Geometry check sheet. Reference: the model listing, model coordinates, mm. A direction names the side the tool comes from. Coordinates: 2 decimals unless noted, no trailing zeros. Write each loop counter-clockwise with the first axis right and the second up, starting at its lowest first coordinate (ties: lowest second). Pieces come first, ordered by that corner, then holes. Notation, with made-up numbers: (26.5, 34.25) -> (30.5, 34.25) arc R10 cw to (30.5, 39.25) -> close; hole circle Ø11 at (60.5, -10). An arc over 180 degrees is marked (long way). Answer in a Markdown table with one row per item. Add a question column.
1. Cross-section at D-D on z = -115. Record the cut outline in (x, y), and give its area (3 significant figures).
2. Mould release check, pull along X, two halves, no side actions. Record for faces 6 (the cylindrical face through (17.27, 0.2, -10.09)), 7 (the flat face through (50.411, 0.197, 33.724)), 8 (the flat face through (-54.411, 0.197, 26.796)): pulls with the +X half, pulls with the -X half, needs draft (parallel to the pull), parting line crosses it, or undercut.
3. Set-up check for faces 1 (the cylindrical face through (-0.49, 0.2, -129.99)), 2 (the flat face through (-51.06, 0.2, 34.1)), 3 (the cylindrical face through (-6.355, 0.203, -23.574)), 4 (the cylindrical face through (-23.762, 0.203, 6.527)), 5 (the cylindrical face through (5.805, 0.203, -96.985)): record each of +Z, -Z, +X, -X, +Y, -Y from which the full face is reachable in a straight line by a thin tool's end or side.
4. Cross-section at C-C on x = 0. Record the cut outline in (y, z), and give its area (3 significant figures).
5. Cross-section at A-A on z = 52.5. Record the cut outline in (x, y).
6. Scan lines: L1, parallel to X at y = 0.05, z = -88; L2, parallel to X at y = 0.15, z = 47; L3, parallel to X at y = 0.1, z = 48.5. Record each from-to range of solid material in increasing order. Write a range as from..to.
7. Cross-section at B-B on y = 0.3. Record the cut outline in (x, z), and give its area (3 significant figures).
Autodesk Fusion 360 part; units mm, degrees
sketch "Sketch1" plane through (0, 0, 0) normal (0, 1, 0) x (1, 0, 0)
  line L0 (0, 130) -> (-112.5833, -65) construction
  line L1 (-112.5833, -65) -> (112.5833, -65) construction
  line L2 (112.5833, -65) -> (0, 130) construction
  line L3 (0, 0) -> (0, 130) construction
  line L4 (0, 0) -> (-112.5833, -65) construction
  line L5 (0, 0) -> (112.5833, -65) construction
  circle A0 centre (0, 115) radius 15
  circle A1 centre (-99.5929, -57.5) radius 15
  circle A2 centre (99.5929, -57.5) radius 15
  circle A3 centre (0, 0) radius 20
  line L6 (-4, 19.5959) -> (4, 19.5959) construction
  line L7 (4, 19.5959) -> (4, 100.5432)
  line L8 (4, 100.5432) -> (-4, 100.5432) construction
  line L9 (-4, 100.5432) -> (-4, 19.5959)
  line L10 (-85.0729, -53.7357) -> (-14.9706, -13.2621)
  line L11 (-18.9706, -6.3339) -> (-89.0729, -46.8075)
  line L12 (89.0729, -46.8075) -> (18.9706, -6.3339)
  line L13 (14.9706, -13.2621) -> (85.0729, -53.7357)
  point P0 (0, 100.5432)
  point P1 (0, 19.5959)
  dimension "d1" = 130
  dimension "d2" = 30
  dimension "d4" = 360
  dimension "d5" = 40
  dimension "d6" = 8
  dimension "d8" = 360
extrude "Extrude1" add sketch "Sketch1" along normal blind 0.4
fillet "Fillet1" radius 24 12 edges at (-4, 0.2, -100.5432) (4, 0.2, -100.5432) (-4, 0.2, -19.5959) (4, 0.2, -19.5959) (-18.9706, 0.2, 6.3339) (-14.9706, 0.2, 13.2621) (14.9706, 0.2, 13.2621) (18.9706, 0.2, 6.3339) (85.0729, 0.2, 53.7357) (89.0729, 0.2, 46.8075) (-89.0729, 0.2, 46.8075) (-85.0729, 0.2, 53.7357)
Results found:
| question | item | result |
|---|---|---|
| 1 | outline | (-15, 0) -> (15, 0) -> (15, 0.4) -> (-15, 0.4) -> close |
| 1 | area | 12.0 mm^2 |
| 2 | face 6 | pulls with the +X half |
| 2 | face 7 | undercut |
| 2 | face 8 | pulls with the -X half |
| 3 | face 1 | +Y, -Y |
| 3 | face 2 | +Z, +Y, -Y |
| 3 | face 3 | -X, +Y, -Y |
| 3 | face 4 | -Z, -X, +Y, -Y |
| 3 | face 5 | +X, +Y, -Y |
| 4 | outline | (0, -130) -> (0.4, -130) -> (0.4, 20) -> (0, 20) -> close |
| 4 | area | 60.0 mm^2 |
| 5 | outline | (-113.74, 0) -> (-80.26, 0) -> (-80.26, 0.4) -> (-113.74, 0.4) -> close; (80.26, 0) -> (113.74, 0) -> (113.74, 0.4) -> (80.26, 0.4) -> close |
| 6 | L1 | x = -4..4 |
| 6 | L2 | x = -110.31..-73.41, 73.41..110.31 |
| 6 | L3 | x = -111.59..-75.83, 75.83..111.59 |
| 7 | outline | (-95.93, 42.95) arc R24 cw to (-78.08, 40.46) -> (-31.39, 13.51) arc R24 cw to (-19.72, -3.31) arc R20 ccw to (-12.73, -15.43) arc R24 cw to (-4, -33.94) -> (-4, -87.85) arc R24 cw to (-10.77, -104.56) arc R15 ccw (long way) to (10.77, -104.56) arc R24 cw to (4, -87.85) -> (4, -33.94) arc R24 cw to (12.73, -15.43) arc R20 ccw to (19.72, -3.31) arc R24 cw to (31.39, 13.51) -> (78.08, 40.46) arc R24 cw to (95.93, 42.95) arc R15 ccw (long way) to (85.17, 61.61) arc R24 cw to (74.08, 47.39) -> (27.39, 20.43) arc R24 cw to (7, 18.74) arc R20 ccw to (-7, 18.74) arc R24 cw to (-27.39, 20.43) -> (-74.08, 47.39) arc R24 cw to (-85.17, 61.61) arc R15 ccw (long way) to start |
| 7 | area | 5,580 mm^2 |
